```python
from build123d import *

# Parameters (mm, degrees)
SKETCH_1_W      = 144
SKETCH_1_H      = 104
SKETCH_1_R      = 1.5
SKETCH_1_W_2    = 133.2
SKETCH_1_H_2    = 79.8
EXTRUDE_1_DEPTH = 1.6
SKETCH_2_W      = 133.2
SKETCH_2_H      = 79.8
EXTRUDE_2_DEPTH = 9.3


with BuildPart() as part:
    # 草图1 → 拉伸1 (new body)
    with BuildSketch(Plane.XY):
        Rectangle(SKETCH_1_W, SKETCH_1_H)
        with Locations((-69, -48.5)):
            Circle(SKETCH_1_R, mode=Mode.SUBTRACT)
        with Locations((-69, 48.5)):
            Circle(SKETCH_1_R, mode=Mode.SUBTRACT)
        with Locations((69, 48.5)):
            Circle(SKETCH_1_R, mode=Mode.SUBTRACT)
        with Locations((69, -48.5)):
            Circle(SKETCH_1_R, mode=Mode.SUBTRACT)
        with Locations((0, 3)):
            Rectangle(SKETCH_1_W_2, SKETCH_1_H_2, mode=Mode.SUBTRACT)
    extrude(amount=EXTRUDE_1_DEPTH)

    # 草图2 → 拉伸2 (add)
    with BuildSketch(Plane(origin=(0, 0, 0), x_dir=(-1, 0, 0), z_dir=(0, 0, -1))):
        with Locations((0, 3)):
            Rectangle(SKETCH_2_W, SKETCH_2_H)
    extrude(amount=-EXTRUDE_2_DEPTH)


solid = part.part
```
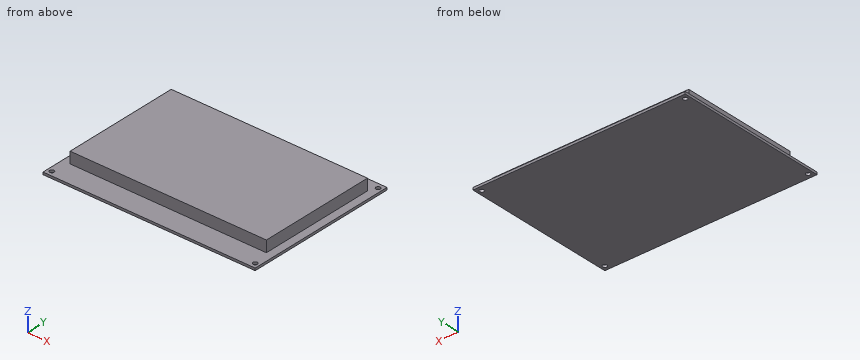
For this review, take the finished solid that the model builds, in its own axes (mm). Give positions to 0.01 mm unless a question says otherwise; leave off trailing zeros. Write each loop counter-clockwise with the first axis right and the second up, starting at its lowest first coordinate (ties: lowest second). Pieces come first, ordered by that corner, then holes.
Item 1: Take a section at B-B (x = 69). Give the boundary of the cut face in (y, z), and give its area (3 significant figures).
Item 2: Wall thickness on probe 1 along Y at (x, z) = (69, 1.2); probe 2 along X at (y, z) = (-18, 2.5); probe 3 along Y at (x, z) = (39, 5.5): over which ranges is each line inside the solid? List them lowest first.
Item 3: Insertion check: P1, Ø2, axis at x = 28.5, z = 8.5, coming from the -Y side; P2, Ø2.5, axis at x = 19.5, z = 3.5, coming from the +Y side; P3, Ø1.8, axis at x = 69, y = 48.5, coming from the +Z side (3 decimals); P4, Ø4, axis at y = 5.5, z = 5, coming from the +X side. Each pin has a flat end and moves straight along its axis. Give the tip position at first contact, or say it passes through.
Item 4: Take a section at C-C (y = 10.5). Give the boundary of the cut face in (x, z), and give its area (3 significant figures).
Item 5: Take a section at A-A (y = 48.5). Give the boundary of the cut face in (x, z), and give its area (3 significant figures).
Item 6: Take a section at D-D (x = 54). Give the boundary of the cut face in (y, z).
Established:
1. outline: (-52, 0) - (-50, 0) - (-50, 1.6) - (-52, 1.6) - close; (-47, 0) - (47, 0) - (47, 1.6) - (-47, 1.6) - close; (50, 0) - (52, 0) - (52, 1.6) - (50, 1.6) - close
1. area: 157 mm2
2. probe 1: y = -52 to -50, -47 to 47, 50 to 52
2. probe 2: x = -66.6 to 66.6
2. probe 3: y = -36.9 to 42.9
3. P1: stops at y = -36.9
3. P2: stops at y = 42.9
3. P3: passes through
3. P4: stops at x = 66.6
4. outline: (-72, 0) - (72, 0) - (72, 1.6) - (66.6, 1.6) - (66.6, 9.3) - (-66.6, 9.3) - (-66.6, 1.6) - (-72, 1.6) - close
4. area: 1,260 mm2
5. outline: (-72, 0) - (-70.5, 0) - (-70.5, 1.6) - (-72, 1.6) - close; (-67.5, 0) - (67.5, 0) - (67.5, 1.6) - (-67.5, 1.6) - close; (70.5, 0) - (72, 0) - (72, 1.6) - (70.5, 1.6) - close
5. area: 221 mm2
6. outline: (-52, 0) - (52, 0) - (52, 1.6) - (42.9, 1.6) - (42.9, 9.3) - (-36.9, 9.3) - (-36.9, 1.6) - (-52, 1.6) - close
